from build123d import *

# Parameters (mm, degrees)
SKETCH_1_R         = 10
SKETCH_1_R_2       = 3
EXTRUDE_1_DEPTH    = 3
HOLE_WIZARD_M3_1_D = 2.5


with BuildPart() as part:
    # 草图1 → 凸台-拉伸1 (new body)
    with BuildSketch(Plane.XY):
        Circle(SKETCH_1_R)
        Circle(SKETCH_1_R_2, mode=Mode.SUBTRACT)
    extrude(amount=EXTRUDE_1_DEPTH)

    # M3 螺纹孔1 (through all)
    with Locations(Plane(origin=(0, 7, 3), x_dir=(1, 0, 0), z_dir=(0, 0, 1))):
        with Locations((0, 0), (-7, -7), (0, -14), (7, -7)):
            Hole(HOLE_WIZARD_M3_1_D / 2)


solid = part.part
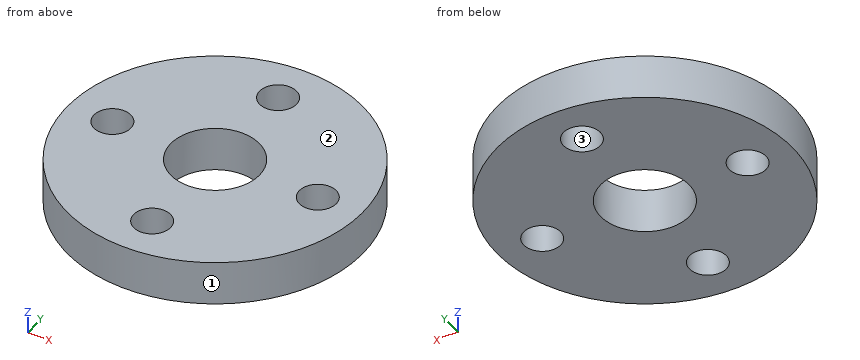
The model under review builds one solid part; all positions refer to its coordinate system, in mm. Face numbers are marked on the shaded views. Round coordinates to 2 decimals unless told otherwise and drop trailing zeros. Order: outer loops, then holes, each group sorted by start corner. A loop starts at its lowest first (then second) coordinate and runs counter-clockwise, first axis right, second up. Notation, with made-up numbers: (35, 22) - (47, 22) arc R18 cw to (47, 46) - close; hole circle Ø5 at (12, 57). An arc over 180 degrees is marked (long way). Use one line per item in the form item = value.
Q1. Add section A-A on y = 0. Give the boundary of the cut face in (x, z).
Response values:
outline = (-10, 0) - (-8.25, 0) - (-8.25, 3) - (-10, 3) - close; (-5.75, 0) - (-3, 0) - (-3, 3) - (-5.75, 3) - close; (3, 0) - (5.75, 0) - (5.75, 3) - (3, 3) - close; (8.25, 0) - (10, 0) - (10, 3) - (8.25, 3) - close
Q2. Add section D-D on z = 1.55. Give the boundary of the cut face in (x, y).
Response values:
outline = circle Ø20 at (0, 0); hole circle Ø2.5 at (-7, 0); hole circle Ø6 at (0, 0); hole circle Ø2.5 at (0, -7); hole circle Ø2.5 at (0, 7); hole circle Ø2.5 at (7, 0)
Q3. Add section C-C on y = -6. Give the boundary of the cut face in (x, z).
Response values:
outline = (-8, 0) - (-0.75, 0) - (-0.75, 3) - (-8, 3) - close; (0.75, 0) - (8, 0) - (8, 3) - (0.75, 3) - close
Q4. Add section B-B on x = 7. Give the boundary of the cut face in (y, z), then the cut area to 3 significant figures.
Response values:
outline = (-7.14, 0) - (-1.25, 0) - (-1.25, 3) - (-7.14, 3) - close; (1.25, 0) - (7.14, 0) - (7.14, 3) - (1.25, 3) - close
area = 35.3 mm^2
Q5. Clearance check with flat-ended pins moving along their axes: P1, Ø1, axis at x = 4, z = 0.5, coming from the -Y side; P2, Ø1.5, axis at y = -5.5, z = 2.5, coming from the -X side; P3, Ø1, axis at x = -3.5, z = 1.5, coming from the +Y side. State where each tip first meets the part, or that it passes through.
Response values:
P1 = -9.37
P2 = -8.8
P3 = 9.54
Q6. To check wall thickness, follow line 1 (Y direction, x = 0, z = 1.85); line 2 (Y direction, x = 0.5, z = 2.05); line 3 (Y direction, x = 8, z = 2.8). State the ranges of each line that lie inside material, in increasing order.
Response values:
line_1 = -10 to -8.25, -5.75 to -3, 3 to 5.75, 8.25 to 10
line_2 = -9.99 to -8.15, -5.85 to -2.96, 2.96 to 5.85, 8.15 to 9.99
line_3 = -6 to -0.75, 0.75 to 6
Q7. Mouldability with a two-part tool opening along X and no side actions: class the marked faces 1, 2 and 3 as pulls with the +X half, pulls with the -X half, needs draft (parallel to the pull), parting line crosses it, or undercut.
Response values:
face_1 = parting line crosses it
face_2 = needs draft
face_3 = undercut
